Geometry: final body of the model. Coordinates: model frame, mm. Give positions to 0.01 mm unless a question says otherwise; leave off trailing zeros. Order: outer loops, then holes, each group sorted by start corner. A loop starts at its lowest first (then second) coordinate and runs counter-clockwise, first axis right, second up. Notation, with made-up numbers: (52, 21.5) -> (90, 21.5) arc R25 cw to (90, 39.5) -> close; hole circle Ø1 at (48, -35). An arc over 180 degrees is marked (long way). Answer in a Markdown table with one row per item. Add a question column.
Q1. Cut plane C-C on x = 38. Return the cut outline in (y, z).
Q2. Cut plane A-A on z = 0.2. Return the cut outline in (x, y), and give its area (3 significant figures).
Q3. Cut plane B-B on y = -3. Return the cut outline in (x, z).
Q4. Line query: line 1 along X through (y, z) = (0.75, 0.45); line 2 along Y through (x, z) = (-2.5, 0.35). Output: solid intervals per line, ascending. Write a range as from..to.
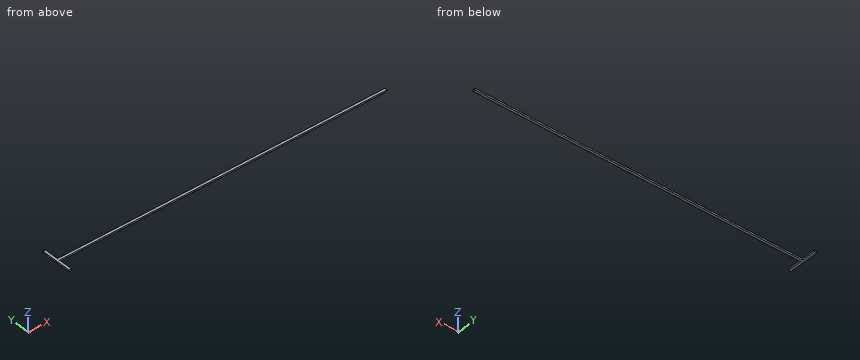
from build123d import *

# Parameters (mm, degrees)
PAD_DEPTH = 0.5


with BuildPart() as part:
    # Sketch → Pad (new body)
    with BuildSketch(Plane.XY):
        Polygon((-7.195606, 5), (-7.195606, 0), (-7.195606, -5), (-6.795606, -5), (-6.395606, -5), (-6.395606, -0.4), (0, -0.4), (100, -0.4), (100, 0.4), (0, 0.4), (-6.395606, 0.4), (-6.395606, 5), (-6.795606, 5), align=None)
    extrude(amount=PAD_DEPTH)


solid = part.part
Completed:
| question | item | result |
|---|---|---|
| 1 | outline | (-0.4, 0) -> (0.4, 0) -> (0.4, 0.5) -> (-0.4, 0.5) -> close |
| 2 | outline | (-7.2, -5) -> (-6.4, -5) -> (-6.4, -0.4) -> (100, -0.4) -> (100, 0.4) -> (-6.4, 0.4) -> (-6.4, 5) -> (-7.2, 5) -> close |
| 2 | area | 93.1 mm² |
| 3 | outline | (-7.2, 0) -> (-6.4, 0) -> (-6.4, 0.5) -> (-7.2, 0.5) -> close |
| 4 | line 1 | x = -7.2..-6.4 |
| 4 | line 2 | y = -0.4..0.4 |
